```python
from build123d import *

# Parameters (mm, degrees)
F0_R     = 16
F0_R_2   = 14
F0_R_3   = 3.15
F1_DEPTH = 4
F2_DEPTH = 3
F3_SIZE  = 3
F4_SIZE  = 1.5


with BuildPart() as f1:
    # F0 (on Top) → F1 (new body)
    with BuildSketch(Plane.XY):
        Circle(F0_R)
        Circle(F0_R_2, mode=Mode.SUBTRACT)
        Circle(F0_R_2)
        Circle(F0_R_3, mode=Mode.SUBTRACT)
    extrude(amount=F1_DEPTH)

    # F0 (on Top) → F2 (join)
    with BuildSketch(Plane.XY):
        Circle(F0_R_2)
        Circle(F0_R_3, mode=Mode.SUBTRACT)
    extrude(amount=-F2_DEPTH)

    # F3
    f3_edges = [f1.edges().sort_by_distance(p)[0] for p in [
        (-3.15, 0, 4),
    ]]
    chamfer(f3_edges, length=F3_SIZE)

    # F4
    f4_edges = [f1.edges().sort_by_distance(p)[0] for p in [
        (-16, 0, 4),
    ]]
    chamfer(f4_edges, length=F4_SIZE)


solid = f1.part
```
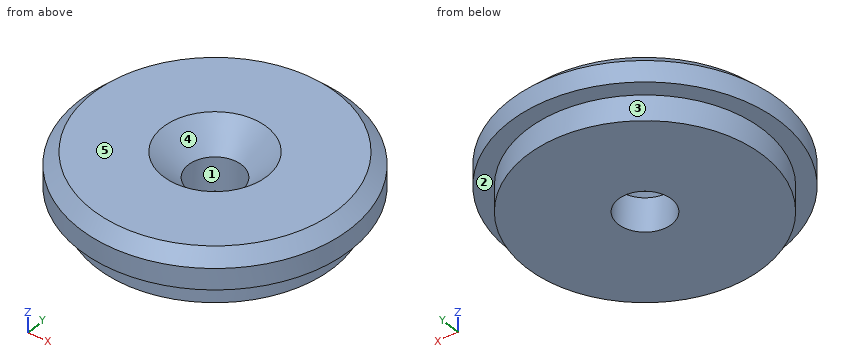
The model under review builds one solid part; all positions refer to its coordinate system, in mm. Face numbers are marked on the shaded views. A direction names the side the tool comes from. Give positions to 0.01 mm unless a question says otherwise; leave off trailing zeros. Write each loop counter-clockwise with the first axis right and the second up, starting at its lowest first coordinate (ties: lowest second). Pieces come first, ordered by that corner, then holes. Notation, with made-up numbers: (65, 77) -> (121, 77) arc R29 cw to (121, 107) -> close; hole circle Ø11 at (-4, -39). An arc over 180 degrees is marked (long way). Put each result on its own line as item: value.
(1) Tool access review of the marked faces 1 and 2: name each direction out of +Z, -Z, +X, -X, +Y, -Y from which nothing blocks a thin tool from reaching the whole face with its end or side.
Results are:
face 1: +Z, -Z
face 2: -Z
(2) For pin 1 Ø5.5 at (x, y) = (0, 0) entering from -Z; pin 2 Ø3 at (x, z) = (-2.5, 1.5) entering from +Y; pin 3 Ø3 at (x, z) = (9.5, 1.5) entering from +Y, all flat-tipped, find the tip position at first contact; note any pin that passes through.
Results are:
pin 1: through
pin 2: y = 15.97
pin 3: y = 13.86
(3) We need section A-A, the plane y = 0. Give the boundary of the cut face in (x, z), and give its area (3 significant figures).
Results are:
outline: (-16, 0) -> (-14, 0) -> (-14, -3) -> (-3.15, -3) -> (-3.15, 1) -> (-6.15, 4) -> (-14.5, 4) -> (-16, 2.5) -> close; (3.15, -3) -> (14, -3) -> (14, 0) -> (16, 0) -> (16, 2.5) -> (14.5, 4) -> (6.15, 4) -> (3.15, 1) -> close
area: 157 mm²
(4) We need section C-C, the plane z = 1.5. Give the boundary of the cut face in (x, y).
Results are:
outline: circle Ø32 at (0, 0); hole circle Ø7.3 at (0, 0)
(5) To check wall thickness, follow probe 1 along Y at (x, z) = (0, -0.9); probe 2 along Y at (x, z) = (0, 0.1); probe 3 along X at (y, z) = (3.5, 2.25). State the ranges of each line that lie inside material, in increasing order. Write a range as from..to.
Results are:
probe 1: -14..-3.15, 3.15..14
probe 2: -16..-3.15, 3.15..16
probe 3: -15.61..-2.67, 2.67..15.61
(6) The part is to be moulded in two halves that separate along Y. For the marked faces 3, 4 and 5, say which applies: pulls with the +Y half, pulls with the -Y half, needs draft (parallel to the pull), parting line crosses it, or undercut.
Results are:
face 3: parting line crosses it
face 4: undercut
face 5: needs draft
